Here's how the part is built. I have some questions about the finished solid (model axes, mm). A direction names the side the tool comes from. Coordinates: 2 decimals unless noted, no trailing zeros. Loops run counter-clockwise (first coordinate to the right, second up) from the corner with the lowest first, then second, coordinate; pieces in that order, holes last. Notation, with made-up numbers: (34.25, 86.25) -> (64.25, 86.25) arc R14 cw to (64.25, 111.25) -> close; hole circle Ø3 at (81, -32). An arc over 180 degrees is marked (long way). Use CSV: the item, a comma, the result in double quotes. Start each with the question number.
from build123d import *

# Parameters (mm, degrees)
F1_DEPTH = 25
F2_DEPTH = 0.6
F3_R     = 0.5


with BuildPart() as f1:
    # F0 (on Top) → F1 (new body)
    with BuildSketch(Plane.XY):
        with BuildLine():
            ThreePointArc((0, -7), (-7, 0), (0, 7))
            Line((0, 7), (2.4, 7))
            ThreePointArc((2.4, 7), (1.2165525061, 7.2993150364), (0, 7.4))
            ThreePointArc((0, 7.4), (-7.4, 0), (0, -7.4))
            ThreePointArc((0, -7.4), (1.2165525061, -7.2993150364), (2.4, -7))
            Line((2.4, -7), (0, -7))
        make_face()
        with BuildLine():
            ThreePointArc((0, 7.4), (1.2165525061, 7.2993150364), (2.4, 7))
            Line((2.4, 7), (11.6, 7))
            ThreePointArc((11.6, 7), (12.7834474939, 7.2993150364), (14, 7.4))
            Line((14, 7.4), (0, 7.4))
        make_face()
        with BuildLine():
            ThreePointArc((14, 7.4), (12.7834474939, 7.2993150364), (11.6, 7))
            Line((11.6, 7), (14, 7))
            ThreePointArc((14, 7), (18.9497474683, 4.9497474683), (21, 0))
            ThreePointArc((21, 0), (18.9497474683, -4.9497474683), (14, -7))
            Line((14, -7), (11.6, -7))
            ThreePointArc((11.6, -7), (12.7834474939, -7.2993150364), (14, -7.4))
            ThreePointArc((14, -7.4), (19.2325901808, -5.2325901808), (21.4, 0))
            ThreePointArc((21.4, 0), (19.2325901808, 5.2325901808), (14, 7.4))
        make_face()
        with BuildLine():
            Line((11.6, -7), (2.4, -7))
            ThreePointArc((2.4, -7), (1.2165525061, -7.2993150364), (0, -7.4))
            Line((0, -7.4), (14, -7.4))
            ThreePointArc((14, -7.4), (12.7834474939, -7.2993150364), (11.6, -7))
        make_face()
    extrude(amount=F1_DEPTH)

    # F0 (on Top) → F2 (join)
    with BuildSketch(Plane.XY):
        with BuildLine():
            ThreePointArc((6.7942857143, 1.6845419652), (4.3132473986, 5.5132473986), (0, 7))
            ThreePointArc((0, 7), (-7, 0), (0, -7))
            ThreePointArc((0, -7), (4.3132473986, -5.5132473986), (6.7942857143, -1.6845419652))
            ThreePointArc((6.7942857143, -1.6845419652), (6.6, 0), (6.7942857143, 1.6845419652))
        make_face()
        with BuildLine():
            ThreePointArc((7, -2.4), (5.2325901808, -5.2325901808), (2.4, -7))
            Line((2.4, -7), (11.6, -7))
            ThreePointArc((11.6, -7), (8.7674098192, -5.2325901808), (7, -2.4))
        make_face()
        with BuildLine():
            ThreePointArc((14, 7), (9.6867526014, 5.5132473986), (7.2057142857, 1.6845419652))
            ThreePointArc((7.2057142857, 1.6845419652), (7.3512681122, 0.8478544349), (7.4, 0))
            ThreePointArc((7.4, 0), (7.3512681122, -0.8478544349), (7.2057142857, -1.6845419652))
            ThreePointArc((7.2057142857, -1.6845419652), (9.6867526014, -5.5132473986), (14, -7))
            ThreePointArc((14, -7), (18.9497474683, -4.9497474683), (21, 0))
            ThreePointArc((21, 0), (18.9497474683, 4.9497474683), (14, 7))
        make_face()
        with BuildLine():
            ThreePointArc((6.7942857143, -1.6845419652), (4.3132473986, -5.5132473986), (0, -7))
            Line((0, -7), (2.4, -7))
            ThreePointArc((2.4, -7), (5.2325901808, -5.2325901808), (7, -2.4))
            ThreePointArc((7, -2.4), (6.8881402122, -2.044859496), (6.7942857143, -1.6845419652))
        make_face()
        with BuildLine():
            ThreePointArc((7.2057142857, -1.6845419652), (7.1118597878, -2.044859496), (7, -2.4))
            ThreePointArc((7, -2.4), (8.7674098192, -5.2325901808), (11.6, -7))
            Line((11.6, -7), (14, -7))
            ThreePointArc((14, -7), (9.6867526014, -5.5132473986), (7.2057142857, -1.6845419652))
        make_face()
        with BuildLine():
            ThreePointArc((7, 0), (6.9483811064, -0.8485281374), (6.7942857143, -1.6845419652))
            ThreePointArc((6.7942857143, -1.6845419652), (6.8881402122, -2.044859496), (7, -2.4))
            ThreePointArc((7, -2.4), (7.1118597878, -2.044859496), (7.2057142857, -1.6845419652))
            ThreePointArc((7.2057142857, -1.6845419652), (7.0516188936, -0.8485281374), (7, 0))
        make_face()
        with BuildLine():
            ThreePointArc((7.2057142857, 1.6845419652), (7.0516188936, 0.8485281374), (7, 0))
            ThreePointArc((7, 0), (7.0516188936, -0.8485281374), (7.2057142857, -1.6845419652))
            ThreePointArc((7.2057142857, -1.6845419652), (7.3512681122, -0.8478544349), (7.4, 0))
            ThreePointArc((7.4, 0), (7.3512681122, 0.8478544349), (7.2057142857, 1.6845419652))
        make_face()
        with BuildLine():
            ThreePointArc((7, 0), (6.9483811064, 0.8485281374), (6.7942857143, 1.6845419652))
            ThreePointArc((6.7942857143, 1.6845419652), (6.6, 0), (6.7942857143, -1.6845419652))
            ThreePointArc((6.7942857143, -1.6845419652), (6.9483811064, -0.8485281374), (7, 0))
        make_face()
        with BuildLine():
            Line((2.4, 7), (0, 7))
            ThreePointArc((0, 7), (4.3132473986, 5.5132473986), (6.7942857143, 1.6845419652))
            ThreePointArc((6.7942857143, 1.6845419652), (6.8881402122, 2.044859496), (7, 2.4))
            ThreePointArc((7, 2.4), (5.2325901808, 5.2325901808), (2.4, 7))
        make_face()
        with BuildLine():
            ThreePointArc((11.6, 7), (8.7674098192, 5.2325901808), (7, 2.4))
            ThreePointArc((7, 2.4), (7.1118597878, 2.044859496), (7.2057142857, 1.6845419652))
            ThreePointArc((7.2057142857, 1.6845419652), (9.6867526014, 5.5132473986), (14, 7))
            Line((14, 7), (11.6, 7))
        make_face()
        with BuildLine():
            ThreePointArc((7, 2.4), (6.8881402122, 2.044859496), (6.7942857143, 1.6845419652))
            ThreePointArc((6.7942857143, 1.6845419652), (6.9483811064, 0.8485281374), (7, 0))
            ThreePointArc((7, 0), (7.0516188936, 0.8485281374), (7.2057142857, 1.6845419652))
            ThreePointArc((7.2057142857, 1.6845419652), (7.1118597878, 2.044859496), (7, 2.4))
        make_face()
        with BuildLine():
            Line((11.6, 7), (2.4, 7))
            ThreePointArc((2.4, 7), (5.2325901808, 5.2325901808), (7, 2.4))
            ThreePointArc((7, 2.4), (8.7674098192, 5.2325901808), (11.6, 7))
        make_face()
    extrude(amount=F2_DEPTH)

    # F3
    f3_edges = [f1.edges().sort_by_distance(p)[0] for p in [
        (-7, 0, 0.6),
        (7, -7, 0.6),
        (21, 0, 0.6),
        (7, 7, 0.6),
    ]]
    fillet(f3_edges, radius=F3_R)


solid = f1.part
1) I want a section at A-A, the plane z = 16.5. Please give me the cut outline in (x, y).
2) Thinking about a two-plate mould opening in X: for faces 1 (the face through (-7.4, 0.16, 12.32)), 2 (the face through (7, -7, 13)), 3 (the face through (7, 7, 13)), 4 (the face through (5.9, 7.2, 25)), which applies, pulls with the +X half, pulls with the -X half, needs draft (parallel to the pull), parting line crosses it, or undercut?
3) Which directions (+Z, -Z, +X, -X, +Y, -Y) give clear straight access to the entire face, cutting with the end or side of a thin tool? Please do faces 5 (the face through (7, 7.4, 12)), 6 (the face through (7, 0, 0.6)).
4) I want a section at B-B, the plane x = 5.5. Please give me the cut outline in (y, z).
5) For P1, Ø2, axis at y = -5, z = 9.5, coming from the -X side; P2, Ø1.5, axis at x = -2.5, z = 7, coming from the -Y side; P3, Ø6, axis at x = -0.5, y = 2, coming from the +Z side, each with a flat end and sliding along its axis, tell me the tip position at first contact or that it passes through.
6) Please list where these lines run through material, in increasing order: L1, parallel to Y at x = -0.25, z = 7; L2, parallel to Z at x = -2.25, y = 4.5; L3, parallel to X at y = -4.75, z = 23. Write a range as [from, to].
Return value:
1,outline,"(0, -7.4) -> (14, -7.4) arc R7.4 ccw to (14, 7.4) -> (0, 7.4) arc R7.4 ccw to start; hole (0, -7) -> (14, -7) arc R7 ccw to (14, 7) -> (0, 7) arc R7 ccw to start"
2,face 1,"pulls with the -X half"
2,face 2,"undercut"
2,face 3,"undercut"
2,face 4,"needs draft"
3,face 5,"+Z, -Z, +X, -X, +Y"
3,face 6,"+Z"
4,outline,"(-7.4, 0) -> (7.4, 0) -> (7.4, 25) -> (7, 25) -> (7, 1.1) arc R0.5 cw to (6.5, 0.6) -> (-6.5, 0.6) arc R0.5 cw to (-7, 1.1) -> (-7, 25) -> (-7.4, 25) -> close"
5,P1,"stops at x = -6.23"
5,P2,"stops at y = -7.19"
5,P3,"stops at z = 0.6"
6,L1,"y = [-7.4, -7], [7, 7.4]"
6,L2,"z = [0, 0.6]"
6,L3,"x = [-5.67, -5.14], [19.14, 19.67]"
